The model under review builds one solid part; all positions refer to its coordinate system, in mm. Give positions to 0.01 mm unless a question says otherwise; leave off trailing zeros. Write each loop counter-clockwise with the first axis right and the second up, starting at its lowest first coordinate (ties: lowest second). Pieces come first, ordered by that corner, then holes. Notation, with made-up numbers: (60.5, 66) - (98.5, 66) arc R17 ccw to (98.5, 76) - close; hole circle Ø8 at (62.25, 64). An arc over 180 degrees is marked (long way). One line per question, with ' | ' between items. Start each with the question number.
```python
from build123d import *

# Parameters (mm, degrees)
SKETCH1_R           = 1.5875
BOSS_EXTRUDE1_DEPTH = 0.79375


with BuildPart() as part:
    # Sketch1 → Boss-Extrude1 (new, symmetric)
    with BuildSketch(Plane(origin=(0, 0, 0), x_dir=(1, 0, 0), z_dir=(0, 1, 0))):
        with BuildLine():
            Line((28, 4.15), (8, 4.15))
            Line((8, 4.15), (-23.85, 4.15))
            ThreePointArc((-23.85, 4.15), (-28, 0), (-23.85, -4.15))
            Line((-23.85, -4.15), (8, -4.15))
            Line((8, -4.15), (28, -4.15))
            ThreePointArc((28, -4.15), (32.15, 0), (28, 4.15))
        make_face()
        with Locations(Location((8, 0, 0), (0, 0, 270))):
            Circle(SKETCH1_R, mode=Mode.SUBTRACT)
        with Locations(Location((28, 0, 0), (0, 0, 270))):
            Circle(SKETCH1_R, mode=Mode.SUBTRACT)
    extrude(amount=BOSS_EXTRUDE1_DEPTH, both=True)


solid = part.part
```
Item 1: Take a section at C-C (y = -0.2). State how many separate pieces and enclosed holes the cut face has, plus the area to 3 significant figures.
Item 2: Take a section at A-A (z = 0). Give the boundary of the cut face in (x, y).
Item 3: For probe 1 along X at (y, z) = (-0.35, 0); probe 2 along X at (y, z) = (0.75, -0.5); probe 3 along Z at (x, y) = (-24, -0.45), list the stretches that pass through material, from the lowest coordinate up.
Item 4: Take a section at D-D (z = 2.5). Give the boundary of the cut face in (x, y).
Item 5: Take a section at B-B (x = 8). Give the boundary of the cut face in (y, z).
Item 6: The part is to be moulded in two halves that separate along X. For faces 1 (the cylindrical face through (9.574, -0.011, -0.207)), 2 (the flat face through (2, 0, -4.15)), 3 (the cylindrical face through (32.15, 0.01, 0.09)), 4 (the cylindrical face through (-28, 0, 0)), say which applies: +X half, -X half, draft (parallel to the pull), parting line (faces both ways), or undercut.
Check sheet entries:
1) separate pieces: 1 | enclosed holes: 2 | area: 469 mm^2
2) outline: (-28, -0.79) - (6.41, -0.79) - (6.41, 0.79) - (-28, 0.79) - close; (9.59, -0.79) - (26.41, -0.79) - (26.41, 0.79) - (9.59, 0.79) - close; (29.59, -0.79) - (32.15, -0.79) - (32.15, 0.79) - (29.59, 0.79) - close
3) probe 1: x = -28 to 6.41, 9.59 to 26.41, 29.59 to 32.15 | probe 2: x = -27.97 to 6.49, 9.51 to 26.49, 29.51 to 32.12 | probe 3: z = -4.15 to 4.15
4) outline: (-27.16, -0.79) - (31.31, -0.79) - (31.31, 0.79) - (-27.16, 0.79) - close
5) outline: (-0.79, -4.15) - (0.79, -4.15) - (0.79, -1.59) - (-0.79, -1.59) - close; (-0.79, 1.59) - (0.79, 1.59) - (0.79, 4.15) - (-0.79, 4.15) - close
6) face 1: undercut | face 2: draft | face 3: +X half | face 4: -X half
